from build123d import *

# Parameters (mm, degrees)
SKETCH1_R           = 2
SKETCH1_R_2         = 1
BOSS_EXTRUDE1_DEPTH = 1
SKETCH2_R           = 2
BOSS_EXTRUDE2_DEPTH = 0.5
BOSS_EXTRUDE3_DEPTH = 2.5


with BuildPart() as part:
    # Sketch1 → Boss-Extrude1 (new body)
    with BuildSketch(Plane.XY):
        Circle(SKETCH1_R)
        Circle(SKETCH1_R_2, mode=Mode.SUBTRACT)
    extrude(amount=BOSS_EXTRUDE1_DEPTH)

    # Sketch2 → Boss-Extrude2 (add)
    with BuildSketch(Plane.XY.offset(1)):
        Circle(SKETCH2_R)
    extrude(amount=BOSS_EXTRUDE2_DEPTH)

    # Sketch3 → Boss-Extrude3 (add)
    with BuildSketch(Plane.XY.offset(1.5)):
        with BuildLine():
            Line((3.25, -0.968245837), (-3.25, -0.968245837))
            ThreePointArc((-3.25, -0.968245837), (-7, 0), (-3.25, 0.968245837))
            Line((-3.25, 0.968245837), (3.25, 0.968245837))
            ThreePointArc((3.25, 0.968245837), (7, 0), (3.25, -0.968245837))
        make_face()
    extrude(amount=BOSS_EXTRUDE3_DEPTH)


solid = part.part
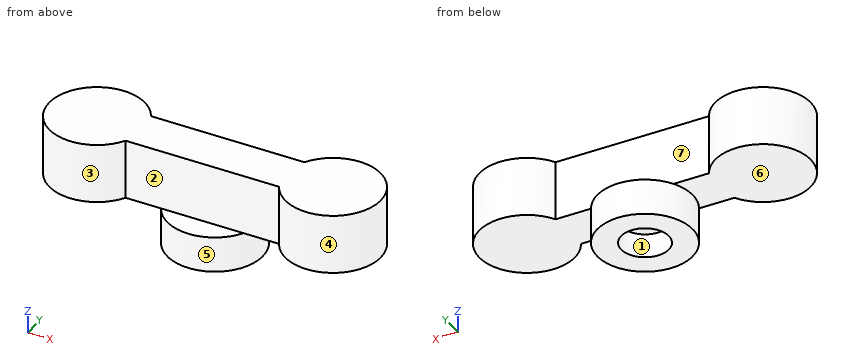
Design review of the part built by this model. Coordinates are the model's own, in mm. Face numbers are marked on the shaded views. A direction names the side the tool comes from. Coordinates: 2 decimals unless noted, no trailing zeros. Write each loop counter-clockwise with the first axis right and the second up, starting at its lowest first coordinate (ties: lowest second). Pieces come first, ordered by that corner, then holes. Notation, with made-up numbers: (-0.5, -20.75) -> (27.5, -20.75) arc R21 ccw to (27.5, -5.75) -> close; hole circle Ø7 at (-3, 4). An arc over 180 degrees is marked (long way). Write each question's results on one line, items separated by ' | '. Start each with the question number.
(1) Take a section at D-D on z = 2.25. Write out the cut boundary in (x, y), and give its area (3 significant figures).
(2) Take a section at A-A on y = -1.2. Write out the cut boundary in (x, z).
(3) The part is to be moulded in two halves that separate along X. For the marked faces 4, 5, 6 and 7, say which applies: pulls with the +X half, pulls with the -X half, needs draft (parallel to the pull), parting line crosses it, or undercut.
(4) For line 1 along Y through (x, z) = (0, 0.55); line 2 along Z through (x, y) = (0, -0.1); line 3 along Z through (x, y) = (4, -1.4), list the stretches that pass through material, from the lowest coordinate up. Write a range as from..to.
(5) Take a section at B-B on x = 0. Write out the cut boundary in (y, z), and give its area (3 significant figures).
(6) Take a section at C-C on y = 0. Write out the cut boundary in (x, z).
(7) Clearance check with flat-ended pins moving along their axes: P1, Ø1.2, axis at x = -0.5, z = 3, coming from the +Y side; P2, Ø0.5, axis at x = 1, y = 1.5, coming from the +Z side; P3, Ø1.5, axis at x = 4, z = 3.5, coming from the -Y side. State where each tip first meets the part, or that it passes through.
(8) Tool access review of the marked faces 1, 2 and 3: name each direction out of +Z, -Z, +X, -X, +Y, -Y from which nothing blocks a thin tool from reaching the whole face with its end or side.
Results found:
1) outline: (-3.25, -0.97) -> (3.25, -0.97) arc R2 ccw (long way) to (3.25, 0.97) -> (-3.25, 0.97) arc R2 ccw (long way) to start | area: 37.1 mm2
2) outline: (-6.6, 1.5) -> (-3.4, 1.5) -> (-3.4, 4) -> (-6.6, 4) -> close; (-1.6, 0) -> (1.6, 0) -> (1.6, 1.5) -> (-1.6, 1.5) -> close; (3.4, 1.5) -> (6.6, 1.5) -> (6.6, 4) -> (3.4, 4) -> close
3) face 4: undercut | face 5: parting line crosses it | face 6: needs draft | face 7: undercut
4) line 1: y = -2..-1, 1..2 | line 2: z = 1..4 | line 3: z = 1.5..4
5) outline: (-2, 0) -> (-1, 0) -> (-1, 1) -> (1, 1) -> (1, 0) -> (2, 0) -> (2, 1.5) -> (0.97, 1.5) -> (0.97, 4) -> (-0.97, 4) -> (-0.97, 1.5) -> (-2, 1.5) -> close | area: 8.84 mm2
6) outline: (-7, 1.5) -> (-2, 1.5) -> (-2, 0) -> (-1, 0) -> (-1, 1) -> (1, 1) -> (1, 0) -> (2, 0) -> (2, 1.5) -> (7, 1.5) -> (7, 4) -> (-7, 4) -> close
7) P1: stops at y = 0.97 | P2: stops at z = 1.5 | P3: stops at y = -1.98
8) face 1: -Z | face 2: +Z, -Y | face 3: +Z, -Z
